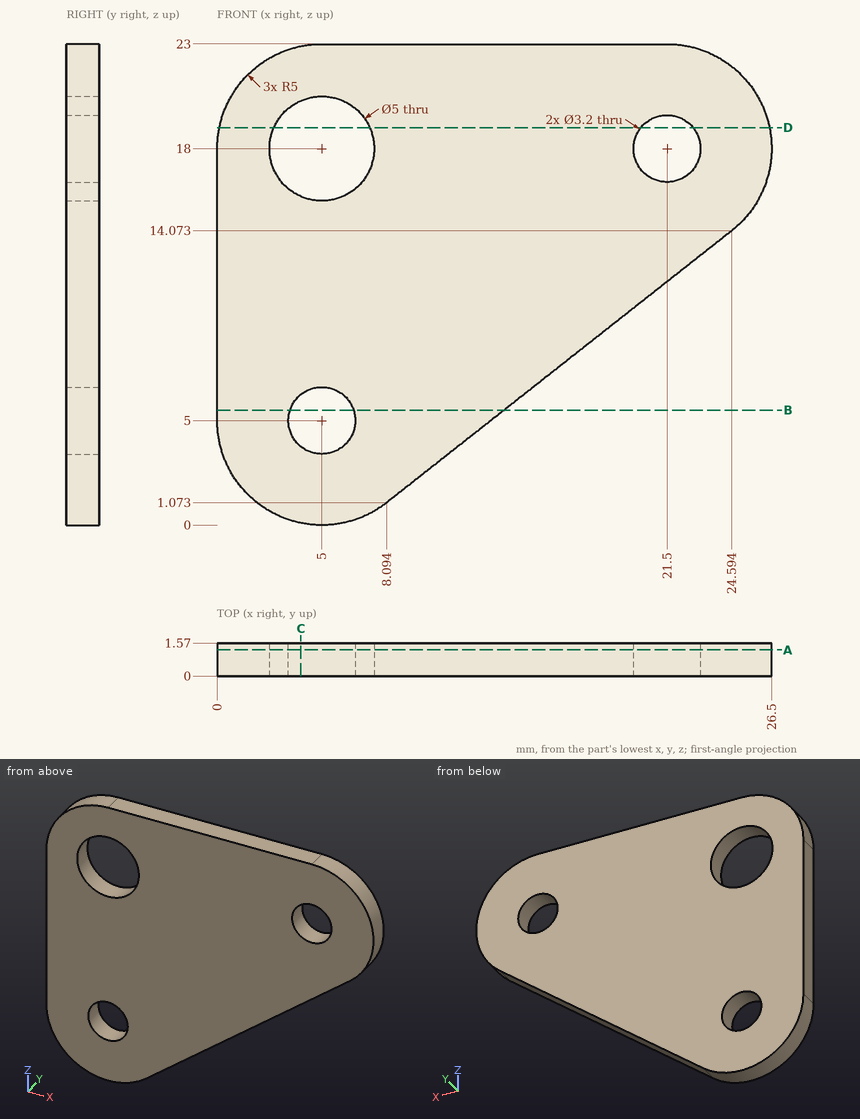
Print and shaded views of the part. All mm, measured from the part's lowest x, y and z. Give positions to 0.01 mm unless a question says otherwise; leave off trailing zeros. Loops run counter-clockwise (first coordinate to the right, second up) from the corner with the lowest first, then second, coordinate; pieces in that order, holes last. Notation, with made-up numbers: (46, -25.75) -> (87, -25.75) arc R26 ccw to (87, 3.25) -> close; hole circle Ø9 at (59, -31). An arc over 180 degrees is marked (long way). One line per question, with ' | ' between items. Start each with the question number.
1) Pin check, flat tip, straight feed: pin 1 (2.5 mm diameter, centred on x = 21.5, z = 18, fed in from -Y). Stop position of the tip, or through.
2) Probe L1, parallel to X at y = 0.8, z = 18; L2, parallel to Z at x = 5, y = 1.15; L3, parallel to Z at x = 6, y = 1.4. List the from-to ranges inside material, lowest first.
3) Cut at B-B (z = 5.5). Give the cut face in (x, y).
4) Cut at D-D (z = 19). Give the cut face in (x, y).
5) Cut at A-A (y = 1.25). Give the cut face in (x, z) (1 decimal).
6) Cut at C-C (x = 4). Give the cut face in (y, z).
Return value:
1) pin 1: through
2) L1: 0 to 2.5, 7.5 to 19.9, 23.1 to 26.5 | L2: 0 to 3.4, 6.6 to 15.5, 20.5 to 23 | L3: 0.1 to 3.75, 6.25 to 15.71, 20.29 to 23
3) outline: (0, 0) -> (3.48, 0) -> (3.48, 1.57) -> (0, 1.57) -> close; (6.52, 0) -> (13.71, 0) -> (13.71, 1.57) -> (6.52, 1.57) -> close
4) outline: (0.1, 0) -> (2.71, 0) -> (2.71, 1.57) -> (0.1, 1.57) -> close; (7.29, 0) -> (20.25, 0) -> (20.25, 1.57) -> (7.29, 1.57) -> close; (22.75, 0) -> (26.4, 0) -> (26.4, 1.57) -> (22.75, 1.57) -> close
5) outline: (0, 5) arc R5 ccw to (8.1, 1.1) -> (24.6, 14.1) arc R5 ccw to (21.5, 23) -> (5, 23) arc R5 ccw to (0, 18) -> close; hole circle Ø5 at (5, 18); hole circle Ø3.2 at (5, 5); hole circle Ø3.2 at (21.5, 18)
6) outline: (0, 0.1) -> (1.57, 0.1) -> (1.57, 3.75) -> (0, 3.75) -> close; (0, 6.25) -> (1.57, 6.25) -> (1.57, 15.71) -> (0, 15.71) -> close; (0, 20.29) -> (1.57, 20.29) -> (1.57, 22.9) -> (0, 22.9) -> close
